The listing builds one solid part. Answer for the finished solid, in the listing's coordinates (mm). A direction names the side the tool comes from. Give positions to 0.01 mm unless a question says otherwise; leave off trailing zeros. Loops run counter-clockwise (first coordinate to the right, second up) from the corner with the lowest first, then second, coordinate; pieces in that order, holes last. Notation, with made-up numbers: (-37, -35.75) - (3, -35.75) arc R29 ccw to (3, -12.75) - close; hole circle Ø8 at (71.25, -7). An arc over 180 degrees is marked (long way). Answer as CSV lines item,"result". Start each with the question number.
1) A cutting plane is placed at D-D (y = 56). Determine the outline of the cut face in (x, z), and give its area (3 significant figures).
2) A cutting plane is placed at C-C (x = 60). Determine the outline of the cut face in (y, z).
3) Flat-ended cylindrical pins translate along their axes: pin 1 (8 mm diameter, centred on x = 40, y = 10, fed in from -Z); pin 2 (2 mm diameter, centred on x = 48.5, z = 5.5, fed in from +Y); pin 3 (6.5 mm diameter, centred on x = 15, y = 42, fed in from +Z); pin 4 (4 mm diameter, centred on y = 59, z = 3, fed in from +X). Find the tip coordinate at first contact, or state that the pin passes through.
4) For faces 4 (the face through (28, 55, 4)), 5 (the face through (5, 55, 4)), 6 (the face through (30.492, 40.304, 5.5)), 7 (the face through (75, 55, 4)), determine the directions among +Z, -Z, +X, -X, +Y, -Y from which every point of the face is accessible in a straight line to the end or side of a thin tool.
5) A cutting plane is placed at B-B (y = 24). Determine the outline of the cut face in (x, z).
6) A cutting plane is placed at A-A (z = 8). Give the number of separate pieces and of enclosed holes in the cut face, and give its area (3 significant figures).
7) Find the intervals of material crossed by line 1 along Y through (x, z) = (60, 3); line 2 along X through (y, z) = (57, 8); line 3 along Y through (x, z) = (20, 4), in increasing order.
8) For a pull along X with two mould halves and no side action, classify faces 1 (the face through (80, 31, 4)), 2 (the face through (2.281, 2.406, 4.563)), 3 (the face through (68.336, 39.587, 4.563)) as pulls with the +X half, pulls with the -X half, needs draft (parallel to the pull), parting line crosses it, or undercut.
```python
from build123d import *

# Parameters (mm, degrees)
ESQUISSE1_W             = 80
ESQUISSE1_H             = 55
BOSS_EXTRU_1_DEPTH      = 9
ESQUISSE2_R             = 11
ESQUISSE2_R_2           = 8.75
ESQUISSE2_R_3           = 1.5
ENL_V_MAT_EXTRU_1_DEPTH = 98.49871794
ESQUISSE3_R             = 3
ENL_V_MAT_EXTRU_2_DEPTH = 98.49871794
CONG_1_R                = 8
BOSS_EXTRU_2_START      = 1.9
ESQUISSE4_R             = 11
ESQUISSE4_R_2           = 9
BOSS_EXTRU_2_DEPTH      = 1.9
ESQUISSE5_W             = 12
ESQUISSE5_H             = 8.5
BOSS_EXTRU_3_DEPTH      = 9


with BuildPart() as part:
    # Esquisse1 → Boss.-Extru.1 (new body)
    with BuildSketch(Plane.XY):
        with Locations((40, 27.5)):
            Rectangle(ESQUISSE1_W, ESQUISSE1_H)
    extrude(amount=BOSS_EXTRU_1_DEPTH)

    # Esquisse2 → Enlèv. mat.-Extru.1 (cut, through all)
    with BuildSketch(Plane.XY.offset(9)):
        with Locations((20, 37)):
            Circle(ESQUISSE2_R)
        with Locations((60, 35)):
            Circle(ESQUISSE2_R_2)
        with Locations((60, 46)):
            Circle(ESQUISSE2_R_3)
        with Locations((69.526279442, 40.5)):
            Circle(ESQUISSE2_R_3)
        with Locations((69.526279442, 29.5)):
            Circle(ESQUISSE2_R_3)
        with Locations((60, 24)):
            Circle(ESQUISSE2_R_3)
        with Locations((50.473720558, 29.5)):
            Circle(ESQUISSE2_R_3)
        with Locations((50.473720558, 40.5)):
            Circle(ESQUISSE2_R_3)
    extrude(amount=-ENL_V_MAT_EXTRU_1_DEPTH, mode=Mode.SUBTRACT)

    # Esquisse3 → Enlèv. mat.-Extru.2 (cut, through all)
    with BuildSketch(Plane.XY.offset(9)):
        with Locations((40, 10)):
            Circle(ESQUISSE3_R)
    extrude(amount=-ENL_V_MAT_EXTRU_2_DEPTH, mode=Mode.SUBTRACT)

    # Congé1
    cong_1_edges = [part.edges().sort_by_distance(p)[0] for p in [
        (80, 0, 4.5),
        (0, 0, 4.5),
    ]]
    fillet(cong_1_edges, radius=CONG_1_R)

    # Esquisse4 → Boss.-Extru.2 (add)
    with BuildSketch(Plane.XY.offset(BOSS_EXTRU_2_START)):
        with Locations((20, 37)):
            Circle(ESQUISSE4_R)
        with Locations(Location((20, 37, 0), (0, 0, 180))):
            Circle(ESQUISSE4_R_2, mode=Mode.SUBTRACT)
    extrude(amount=-BOSS_EXTRU_2_DEPTH)

    # Esquisse5 → Boss.-Extru.3 (add)
    with BuildSketch(Plane.XY.offset(9)):
        with Locations((40, 59.25)):
            Rectangle(ESQUISSE5_W, ESQUISSE5_H)
        with Locations((16, 59.25)):
            Rectangle(ESQUISSE5_W, ESQUISSE5_H)
        with Locations((64, 59.25)):
            Rectangle(ESQUISSE5_W, ESQUISSE5_H)
    extrude(amount=-BOSS_EXTRU_3_DEPTH)


solid = part.part
```
Ans:
1,outline,"(10, 0) - (22, 0) - (22, 9) - (10, 9) - close; (34, 0) - (46, 0) - (46, 9) - (34, 9) - close; (58, 0) - (70, 0) - (70, 9) - (58, 9) - close"
1,area,"324 mm2"
2,outline,"(0, 0) - (22.5, 0) - (22.5, 9) - (0, 9) - close; (25.5, 0) - (26.25, 0) - (26.25, 9) - (25.5, 9) - close; (43.75, 0) - (44.5, 0) - (44.5, 9) - (43.75, 9) - close; (47.5, 0) - (63.5, 0) - (63.5, 9) - (47.5, 9) - close"
3,pin 1,"z = 0"
3,pin 2,"y = 55"
3,pin 3,"z = 1.9"
3,pin 4,"x = 70"
4,face 4,"+Z, -Z, +Y"
4,face 5,"+Z, -Z, -X, +Y"
4,face 6,"+Z"
4,face 7,"+Z, -Z, +X, +Y"
5,outline,"(0, 0) - (58.5, 0) - (58.5, 9) - (0, 9) - close; (61.5, 0) - (80, 0) - (80, 9) - (61.5, 9) - close"
6,separate pieces,"1"
6,enclosed holes,"9"
6,area,"3,990 mm2"
7,line 1,"0 to 22.5, 25.5 to 26.25, 43.75 to 44.5, 47.5 to 63.5"
7,line 2,"10 to 22, 34 to 46, 58 to 70"
7,line 3,"0 to 26, 48 to 63.5"
8,face 1,"pulls with the +X half"
8,face 2,"pulls with the -X half"
8,face 3,"undercut"
